Check sheet for the modelled part. Datum: model origin and axes. Units: mm. A direction names the side the tool comes from. Give positions to 0.01 mm unless a question says otherwise; leave off trailing zeros.
Item 1: Access from +Z, -Z, +X, -X, +Y, -Y to the whole of each face (thin tool, end or side, straight path). Record for faces 5 (the conical face through (4.79, -8.22, -2.12)), 6 (the cylindrical face through (-1.11, -8.452, -0.94)).
Item 2: Release check for a two-part mould opening along X. For faces 1 (the cylindrical face through (4.864, -1.532, -6.571)), 2 (the conical face through (-4.79, 8.22, -2.12)), 3 (the flat face through (-5, 4, -13.3)), 4 (the flat face through (7.83, 4.44, -7.06)) record: released by +X, released by -X, zero draft, split by the parting line, or undercut.
Item 3: Material ranges on line 1 along Y through (x, z) = (0, -7.5); line 2 along X through (y, z) = (2.25, -11.25); line 3 along Y through (x, z) = (4.5, -7), recorded low to high.
from build123d import *

# Parameters (mm, degrees)
CUT_EXTRUDE1_START = -12.602516
SKETCH2_OUTSIDE_W  = 29.232
SKETCH2_OUTSIDE_H  = 29.232
CUT_EXTRUDE1_DEPTH = 11.234893
FILLET1_R          = 0.5


with BuildPart() as part:
    # Sketch1 → Revolve1 (revolve)
    with BuildSketch(Plane(origin=(0, 0, 0), x_dir=(0, 0, -1), z_dir=(1, 0, 0)), mode=Mode.PRIVATE) as revolve1_sk:
        Polygon((13.3, 7.791923789), (13.3, 6.1), (12.3, 5.1), (1, 5.1), (0, 6.1), (0, 8.524769367), (1.367623399, 8.524769367), (1.367623399, 9.162502632), (4, 10.39), (11.8, 10.39), align=None)
    revolve(revolve1_sk.sketch.rotate(Axis((0, 0, 0), (0, 0, -1)), 90), axis=Axis((0, 0, 0), (0, 0, -1)))

    # Sketch2 outside → Cut-Extrude1 (cut)
    with BuildSketch(Plane.XY.offset(CUT_EXTRUDE1_START)):
        Rectangle(SKETCH2_OUTSIDE_W, SKETCH2_OUTSIDE_H)
        Polygon((10.392304845, 0), (5.196152423, 9), (-5.196152423, 9), (-10.392304845, 0), (-5.196152423, -9), (5.196152423, -9), align=None, mode=Mode.SUBTRACT)
    extrude(amount=CUT_EXTRUDE1_DEPTH, mode=Mode.SUBTRACT)

    # Fillet1
    fillet1_edges = [part.edges().sort_by_distance(p)[0] for p in [
        (-8.524769367, 0, 0),
    ]]
    fillet(fillet1_edges, radius=FILLET1_R)


solid = part.part
Report:
1. face 5: +Z, +X, -Y
1. face 6: +Z
2. face 1: undercut
2. face 2: released by -X
2. face 3: zero draft
2. face 4: released by +X
3. line 1: y = -9 to -5.1, 5.1 to 9
3. line 2: x = -9.09 to -4.58, 4.58 to 9.09
3. line 3: y = -9 to -2.4, 2.4 to 9
